Build history of the part. All positions in model axes, mm. A direction names the side the tool comes from. Round coordinates to 2 decimals unless told otherwise and drop trailing zeros. Order: outer loops, then holes, each group sorted by start corner. A loop starts at its lowest first (then second) coordinate and runs counter-clockwise, first axis right, second up. Notation, with made-up numbers: (-19, 56.5) -> (4, 56.5) arc R17 cw to (4, 73.5) -> close; hole circle Ø6 at (-21, 44). An arc over 180 degrees is marked (long way). Answer as a JSON object with one key per item and string values.
from build123d import *

# Parameters (mm, degrees)
SKETCH1_R           = 9
SKETCH1_R_2         = 5
BOSS_EXTRUDE1_DEPTH = 20
SKETCH3_R           = 6.4
BOSS_EXTRUDE2_DEPTH = 50
CUT_EXTRUDE2_DEPTH  = 16
SKETCH1_3_R         = 9
BOSS_EXTRUDE3_DEPTH = 2
SKETCH1_4_R         = 5
BOSS_EXTRUDE4_DEPTH = 2
CUT_EXTRUDE3_DEPTH  = 42
SKETCH10_R          = 4
BOSS_EXTRUDE5_DEPTH = 20


with BuildPart() as part:
    # Sketch1 → Boss-Extrude1 (new body)
    with BuildSketch(Plane.XY):
        Circle(SKETCH1_R)
        Circle(SKETCH1_R_2, mode=Mode.SUBTRACT)
    extrude(amount=BOSS_EXTRUDE1_DEPTH)

    # Sketch3 → Boss-Extrude2 (add)
    with BuildSketch(Plane(origin=(0, 0, 0), x_dir=(-1, 0, 0), z_dir=(0, 0, -1))):
        Circle(SKETCH3_R)
    extrude(amount=BOSS_EXTRUDE2_DEPTH)

    # Sketch8 → Cut-Extrude2 (cut)
    with BuildSketch(Plane.XY.offset(20)):
        Polygon((0, -7), (2.5, -7), (2.5, -4.330127019), (-2.5, -4.330127019), (-2.5, -7), align=None)
    extrude(amount=-CUT_EXTRUDE2_DEPTH, mode=Mode.SUBTRACT)

    # Sketch1_3 → Boss-Extrude3 (add)
    with BuildSketch(Plane.XY):
        Circle(SKETCH1_3_R)
    extrude(amount=-BOSS_EXTRUDE3_DEPTH)

    # Sketch1_4 → Boss-Extrude4 (add)
    with BuildSketch(Plane.XY):
        Circle(SKETCH1_4_R)
    extrude(amount=BOSS_EXTRUDE4_DEPTH)

    # Sketch9 → Cut-Extrude3 (cut)
    with BuildSketch(Plane(origin=(0, 0, -50), x_dir=(-1, 0, 0), z_dir=(0, 0, -1))):
        Polygon((0, 4.9), (2.16, 4.9), (2.16, 6.02448338), (0.743273512, 7.441209868), (-1.718196928, 7.441209868), (-2.16, 6.02448338), (-2.16, 4.9), align=None)
    extrude(amount=-CUT_EXTRUDE3_DEPTH, mode=Mode.SUBTRACT)

    # Sketch10 → Boss-Extrude5 (add)
    with BuildSketch(Plane(origin=(0, 0, -50), x_dir=(-1, 0, 0), z_dir=(0, 0, -1))):
        Circle(SKETCH10_R)
    extrude(amount=BOSS_EXTRUDE5_DEPTH)


solid = part.part
1) Cut at C-C, the plane z = -26. Give the cut face in (x, y), plus the area to 3 significant figures.
Checked values:
{"outline": "(-2.16, 4.9) -> (-2.16, 6.02) arc R6.4 ccw (long way) to (2.16, 6.02) -> (2.16, 4.9) -> close", "area": "123 mm²"}
2) Cut at D-D, the plane z = 1. Give the cut face in (x, y).
Checked values:
{"outline": "circle Ø18 at (0, 0)"}
3) Which spindle directions (+Z, -Z, +X, -X, +Y, -Y) get a long thin tool onto all of the face, cutting with end or side? Do faces 1 (the face through (0, 6, -8)), 2 (the face through (0, 0, -70)), 3 (the face through (0, -7, 12)), 4 (the face through (4, 4, 20)), 5 (the face through (0.867, -3.905, -59.86)). Say none if no direction does.
Checked values:
{"face 1": "-Z, +Y", "face 2": "-Z, +X, -X, +Y, -Y", "face 3": "+Z", "face 4": "+Z, +X, -X, +Y, -Y", "face 5": "-Z"}
4) Flat gauge pins, fed straight in: pin 1 Ø2 at (x, z) = (-5, -26.5) entering from -Y; pin 2 Ø2 at (y, z) = (-6, 14.5) entering from +X; pin 3 Ø0.9 at (y, z) = (5.5, -36) entering from -X. Where does each tip first touch, or does it go through?
Checked values:
{"pin 1": "stops at y = -5", "pin 2": "stops at x = 7.48", "pin 3": "stops at x = -3.93"}
5) Probe L1, parallel to Y at x = 0, z = 7; L2, parallel to Z at x = 0.5, y = 6; L3, parallel to Z at x = -2.25, y = -3.25. List the from-to ranges inside material, lowest first. Write a range as from..to.
Checked values:
{"L1": "y = -9..-7, 5..9", "L2": "z = -8..20", "L3": "z = -70..2"}
6) Cut at A-A, the plane x = 0. Give the cut face in (y, z), plus the area to 3 significant figures.
Checked values:
{"outline": "(-9, -2) -> (-6.4, -2) -> (-6.4, -50) -> (-4, -50) -> (-4, -70) -> (4, -70) -> (4, -50) -> (4.9, -50) -> (4.9, -8) -> (6.4, -8) -> (6.4, -2) -> (9, -2) -> (9, 20) -> (5, 20) -> (5, 2) -> (-5, 2) -> (-5, 4) -> (-7, 4) -> (-7, 20) -> (-9, 20) -> close", "area": "895 mm²"}
7) Cut at B-B, the plane y = 0. Give the cut face in (x, z).
Checked values:
{"outline": "(-9, -2) -> (-6.4, -2) -> (-6.4, -50) -> (-4, -50) -> (-4, -70) -> (4, -70) -> (4, -50) -> (6.4, -50) -> (6.4, -2) -> (9, -2) -> (9, 20) -> (5, 20) -> (5, 2) -> (-5, 2) -> (-5, 20) -> (-9, 20) -> close"}
8) Pull direction Y, two halves, no side cores. Call faces 6 (the face through (-0.651, 4.957, 10.874)), 7 (the face through (-1.172, 8.923, 9.154)), 8 (the face through (0, 4.9, -29)): pulls with the +Y half, pulls with the -Y half, needs draft (parallel to the pull), parting line crosses it, or undercut.
Checked values:
{"face 6": "undercut", "face 7": "parting line crosses it", "face 8": "pulls with the +Y half"}
